Check sheet for the modelled part. Datum: model origin and axes. Units: mm. Face numbers are marked on the shaded views. A direction names the side the tool comes from. Coordinates: 2 decimals unless noted, no trailing zeros. Loops run counter-clockwise (first coordinate to the right, second up) from the corner with the lowest first, then second, coordinate; pieces in that order, holes last. Notation, with made-up numbers: M 12,58.25 L 17,58.25 A24 cw 17,70.25 Z; hole C -33.75,65.5 d6. An arc over 180 degrees is marked long. Answer as CSV lines item,"result". Start each with the question number.
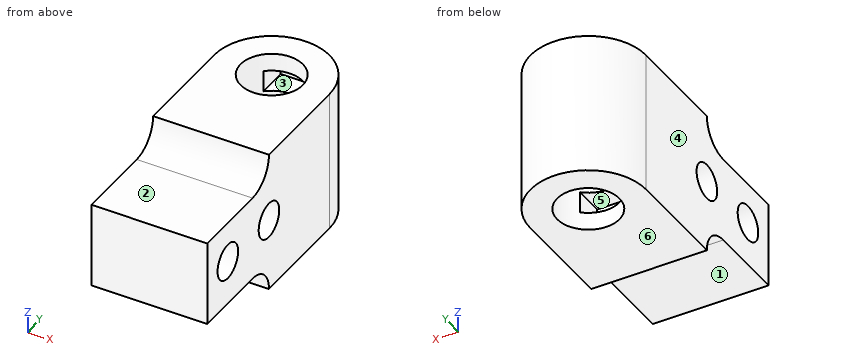
from build123d import *

# Parameters (mm, degrees)
F0_W     = 32.5
F0_H     = 30
F1_DEPTH = 40
F2_R     = 5
F3_DEPTH = 32.5
F4_R     = 8.75
F5_DEPTH = 40
F6_W     = 29.5
F6_H     = 6
F7_DEPTH = 6


with BuildPart() as f1:
    # F0 (on Top) → F1 (new body)
    with BuildSketch(Plane.XY):
        with BuildLine():
            Line((16.25, -29.5), (16.25, 0))
            ThreePointArc((16.25, 0), (0, 16.25), (-16.25, 0))
            Line((-16.25, 0), (-16.25, -29.5))
            Line((-16.25, -29.5), (16.25, -29.5))
        make_face()
        with Locations((0, -44.5)):
            Rectangle(F0_W, F0_H)
    extrude(amount=F1_DEPTH)

    # F2 (on face) → F3 (cut)
    with BuildSketch(Plane(origin=(-16.25, 0, 0), x_dir=(0, -1, 0), z_dir=(-1, 0, 0))):
        with BuildLine():
            Line((37.5, 32), (59.5, 32))
            Line((59.5, 32), (59.5, 40))
            Line((59.5, 40), (29.5, 40))
            ThreePointArc((29.5, 40), (31.843146, 34.343146), (37.5, 32))
        make_face()
        with BuildLine():
            Line((29.5, 0), (59.5, 0))
            Line((59.5, 0), (59.5, 8))
            Line((59.5, 8), (37.5, 8))
            ThreePointArc((37.5, 8), (31.843146, 5.656854), (29.5, 0))
        make_face()
        with Locations((29.5, 20.5)):
            Circle(F2_R)
        with Locations((49.5, 20.5)):
            Circle(F2_R)
    extrude(amount=-F3_DEPTH, mode=Mode.SUBTRACT)

    # F4 (on face) → F5 (cut)
    with BuildSketch(Plane.XY.offset(40)):
        Circle(F4_R)
    extrude(amount=-F5_DEPTH, mode=Mode.SUBTRACT)

    # F6 (on Right) → F7 (cut, symmetric)
    with BuildSketch(Plane.YZ):
        Polygon((-14.75, 29), (14.75, 29), (14.75, 35), (0, 35), (-14.75, 35), align=None)
        with Locations((0, 8)):
            Rectangle(F6_W, F6_H)
    extrude(amount=F7_DEPTH, both=True, mode=Mode.SUBTRACT)


solid = f1.part
Item 1: Sectioned sample at B-B, the plane x = 0. Give the number of separate pieces and of enclosed holes in the cut face, and give its area (3 significant figures).
Item 2: Material ranges on line 1 (Z direction, x = 7, y = -49.5); line 2 (Y direction, x = 1, z = 16); line 3 (Y direction, x = -4.5, z = 18), recorded low to high. Write a range as from..to.
Item 3: Set-up check for the marked faces 1, 2 and 3: record each of +Z, -Z, +X, -X, +Y, -Y from which the full face is reachable in a straight line by a thin tool's end or side.
Item 4: Go/stop test with flat-tipped pins: pin 1 (4 mm diameter, centred on x = -3, z = 22, fed in from +Y); pin 2 (8 mm diameter, centred on y = -29.5, z = 20.5, fed in from +X); pin 3 (6.5 mm diameter, centred on y = 10, z = 32, fed in from +X); pin 4 (12 mm diameter, centred on x = 10.5, z = 24, fed in from +Y). Record where each tip stops, or that it passes through.
Item 5: Release check for a two-part mould opening along X. For the marked faces 4, 5 and 6 record: released by +X, released by -X, zero draft, split by the parting line, or undercut.
Item 6: Sectioned sample at A-A, the plane z = 24.5. Record the boundary of the cut face in (x, y).
Item 7: Sectioned sample at D-D, the plane y = -12.5. Record the boundary of the cut face in (x, z), and give its area (3 significant figures).
Item 8: Sectioned sample at C-C, the plane y = -25.5. Record the boundary of the cut face in (x, z), and give its area (4 significant figures).
Reply:
1,separate pieces,"2"
1,enclosed holes,"2"
1,area,"1,580 mm²"
2,line 1,"8..15.5, 25.5..32"
2,line 2,"-59.5..-51.68, -47.32..-31.68, -27.32..-8.69, 8.69..16.22"
2,line 3,"-59.5..-53.83, -45.17..-33.83, -25.17..-7.5, 7.5..15.61"
3,face 1,"-Z, +X, -X, -Y"
3,face 2,"+Z, +X, -X, -Y"
3,face 3,"none"
4,pin 1,"y = 16.22"
4,pin 2,"through"
4,pin 3,"x = 14.78"
4,pin 4,"y = 15.61"
5,face 4,"released by -X"
5,face 5,"undercut"
5,face 6,"zero draft"
6,outline,"M -16.25,-59.5 L 16.25,-59.5 L 16.25,-52.5 L -16.25,-52.5 Z; M -16.25,-46.5 L 16.25,-46.5 L 16.25,-32.5 L -16.25,-32.5 Z; M -16.25,-26.5 L 16.25,-26.5 L 16.25,0 A16.25 ccw -16.25,0 Z; hole C 0,0 d17.5"
7,outline,"M -16.25,0 L 16.25,0 L 16.25,40 L -16.25,40 Z; hole M -6,5 L 6,5 L 6,11 L -6,11 Z; hole M -6,29 L 6,29 L 6,35 L -6,35 Z"
7,area,"1,160 mm²"
8,outline,"M -16.25,0 L 16.25,0 L 16.25,17.5 L -16.25,17.5 Z; M -16.25,23.5 L 16.25,23.5 L 16.25,40 L -16.25,40 Z"
8,area,"1,105 mm²"
